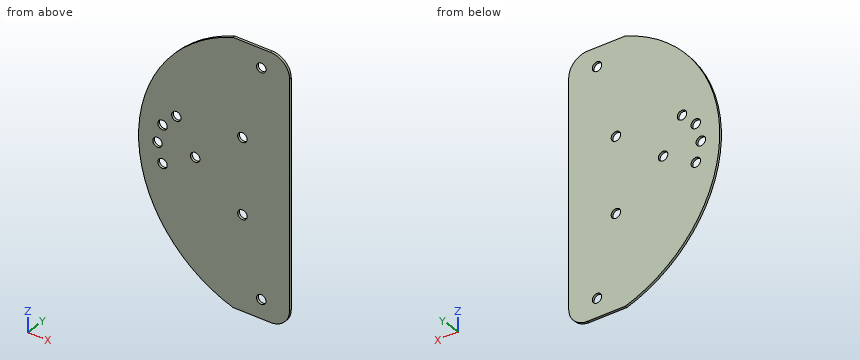
```python
from build123d import *

# Parameters (mm, degrees)
F0_DEPTH = 3.175
F2_D     = 12.7


with BuildPart() as f0:
    # F1 (on Front) → F0 (new body)
    with BuildSketch(Plane.XZ):
        with BuildLine():
            ThreePointArc((-38.1, 177.8), (-165.1, 0), (-38.1, -177.8))
            Line((-38.1, -177.8), (-38.1, 177.8))
        make_face()
        with BuildLine():
            Line((-38.1, 177.8), (-38.1, -177.8))
            Line((-38.1, -177.8), (12.7, -177.8))
            ThreePointArc((12.7, -177.8), (30.6605122421, -170.3605122421), (38.1, -152.4))
            Line((38.1, -152.4), (38.1, 152.4))
            ThreePointArc((38.1, 152.4), (30.6605122421, 170.3605122421), (12.7, 177.8))
            Line((12.7, 177.8), (-38.1, 177.8))
        make_face()
    extrude(amount=F0_DEPTH)

    # F2 (through all)
    with Locations(Plane(origin=(0, 0, 0), x_dir=(1, 0, 0), z_dir=(0, 1, 0))):
        with Locations((-88.9, 0), (-139.7, 0), (0, 152.4), (0, -152.4), (-132.8928, 25.4), (-132.8928, -25.4), (-114.3, -43.9928), (-25.4, -50.8), (-25.4, 50.8)):
            Hole(F2_D / 2)


solid = f0.part
```
Geometry check sheet. Reference: the model listing, model coordinates, mm. Give positions to 0.01 mm unless a question says otherwise; leave off trailing zeros. Write each loop counter-clockwise with the first axis right and the second up, starting at its lowest first coordinate (ties: lowest second). Pieces come first, ordered by that corner, then holes.
1) Section check B-B, the plane z = 25.4. Record the boundary of the cut face in (x, y) (3 decimals), and give its area (3 significant figures).
2) Material ranges on L1, parallel to Z at x = 0, y = -0.85; L2, parallel to Z at x = -138, y = -2.7; L3, parallel to Z at x = -88, y = -2.6, recorded low to high.
3) Gauge pin test, flat ends, axial feed: pin 1 (1 mm diameter, centred on y = -0.5, z = 111.5, fed in from -X); pin 2 (1 mm diameter, centred on x = -95.5, y = -1, fed in from +Z). Record the tip position at first contact, or that the pin passes through.
4) Section check A-A, the plane x = 0. Record the boundary of the cut face in (y, z) (3 decimals), and give its area (3 significant figures).
5) Section check D-D, the plane x = -114.3. Record the boundary of the cut face in (y, z) (3 decimals), and give its area (3 significant figures).
6) Section check C-C, the plane y = -1.4. State how many separate pieces and enclosed holes the cut face has, and give its area (3 significant figures).
Computed:
1. outline: (-163.376, -3.175) - (-139.243, -3.175) - (-139.243, 0) - (-163.376, 0) - close; (-126.543, -3.175) - (38.1, -3.175) - (38.1, 0) - (-126.543, 0) - close
1. area: 599 mm2
2. L1: z = -177.8 to -158.75, -146.05 to 146.05, 158.75 to 177.8
2. L2: z = -97.23 to -29.17, -21.63 to -6.12, 6.12 to 21.63, 29.17 to 97.23
2. L3: z = -151.79 to -6.29, 6.29 to 151.79
3. pin 1: stops at x = -128.82
3. pin 2: stops at z = 146.42
4. outline: (-3.175, -177.8) - (0, -177.8) - (0, -158.75) - (-3.175, -158.75) - close; (-3.175, -146.05) - (0, -146.05) - (0, 146.05) - (-3.175, 146.05) - close; (-3.175, 158.75) - (0, 158.75) - (0, 177.8) - (-3.175, 177.8) - close
4. area: 1,050 mm2
5. outline: (-3.175, -128.515) - (0, -128.515) - (0, 37.643) - (-3.175, 37.643) - close; (-3.175, 50.343) - (0, 50.343) - (0, 128.515) - (-3.175, 128.515) - close
5. area: 776 mm2
6. separate pieces: 1
6. enclosed holes: 9
6. area: 58,700 mm2
